Autodesk Inventor part; units mm, degrees
ref_plane "YZ Plane" through (0, 0, 0) normal (1, 0, 0) x (0, 1, 0)
ref_plane "XZ Plane" through (0, 0, 0) normal (0, 1, 0) x (-1, 0, 0)
ref_plane "XY Plane" through (0, 0, 0) normal (0, 0, 1) x (1, 0, 0)
sketch "Sketch1" plane through (0, 0, 0) normal (0, 0, 1) x (1, 0, 0)
  line L0 (21.2725, 0) -> (23.8125, 0)
  line L1 (23.8125, 0) -> (23.8125, 28.3972)
  line L2 (23.8125, 28.3972) -> (6.985, 28.3972)
  line L3 (21.2725, 25.8572) -> (21.2725, 0)
  line L4 (0, -5.6794) -> (0, 34.0766)
  line L5 (6.985, 25.8572) -> (6.985, 28.3972)
  line L6 (6.985, 25.8572) -> (21.2725, 25.8572)
  point P0 (0, 0)
  dimension "d5" = 28.3972
  dimension "d10" = 21.2725
  dimension "d13" = 2.54
  dimension "d22" = 6.985
  dimension "d50" = 2.54
revolve "Revolution1" add sketch "Sketch1" angle 360 about axis through (0, -10, 0) along (0, 1, 0)
sketch "Sketch4" plane through (0, 0, 0) normal (1, 0, 0) x (0, 1, 0)
  circle A0 centre (8.001, 0) radius 1.5875
  point P0 (0, 0)
  dimension "d33" = 3.175
  dimension "d34" = 8.001
extrude "Extrusion2" cut sketch "Sketch4" along normal through all
pattern_circular "Circular Pattern1" count 3 over 360 about axis through (0, 14.1986, 0) along (0, -1, 0) of "Extrusion2"
sketch "Sketch5" plane through (0, 28.3972, 0) normal (0, 1, 0) x (1, 0, 0)
  line L0 (6.985, 7.9248) -> (-6.985, 7.9248)
  line L1 (-6.985, 7.9248) -> (-6.985, -8.5852)
  line L2 (-6.985, -8.5852) -> (6.985, -8.5852)
  line L3 (6.985, -8.5852) -> (6.985, 7.9248)
  line L4 (6.985, 7.9248) -> (-6.985, -8.5852) construction
  line L5 (-6.985, 7.9248) -> (6.985, -8.5852) construction
  circle A0 centre (0, 0) radius 6.985 construction
  point P0 (0, -0.3302)
  dimension "d51" = 13.97
  dimension "d52" = 16.51
  dimension "d56" = 0.3302
extrude "Extrusion3" cut sketch "Sketch5" against normal through all
sketch "Sketch6" plane through (0, 28.3972, 0) normal (0, 1, 0) x (1, 0, 0)
  circle A0 centre (-15.24, -7.62) radius 1.3959
  line L0 (0, 0) -> (-15.24, -7.62) construction
  line L1 (-15.24, -7.62) -> (0, -7.62) construction
  line L2 (0, -7.62) -> (0, 0) construction
  dimension "d59" = 7.62
  dimension "d60" = 15.24
extrude "Extrusion4" cut sketch "Sketch6" against normal through all
properties part number "Gauge Housing"
Verification items for the finished model (mm, model axes). A direction names the side the tool comes from. Give positions to 0.01 mm unless a question says otherwise; leave off trailing zeros. Order: outer loops, then holes, each group sorted by start corner. A loop starts at its lowest first (then second) coordinate and runs counter-clockwise, first axis right, second up. Notation, with made-up numbers: (2.5, -19.5) -> (30.5, -19.5) arc R28 ccw to (30.5, 11.5) -> close; hole circle Ø10 at (16.25, -32.5). An arc over 180 degrees is marked (long way). Answer as CSV lines item,"result".
Q1. Sectioned sample at B-B on z = 0. Record the cut outline in (x, y) (1 decimal).
Solutions:
outline,"(-23.8, 0) -> (-21.3, 0) -> (-21.3, 25.9) -> (-7, 25.9) -> (-7, 28.4) -> (-23.8, 28.4) -> close; (7, 25.9) -> (21.3, 25.9) -> (21.3, 9.6) -> (23.8, 9.6) -> (23.8, 28.4) -> (7, 28.4) -> close; (21.3, 0) -> (23.8, 0) -> (23.8, 6.4) -> (21.3, 6.4) -> close"
Q2. Release check for a two-part mould opening along Z. For faces 5 (the cylindrical face through (-18.897, 14.397, 14.49)), 6 (the flat face through (-9, 0, -20)), 7 (the cylindrical face through (-16.881, 12.748, -12.944)) record: +Z half, -Z half, draft (parallel to the pull), parting line (faces both ways), or undercut.
Solutions:
face 5,"parting line"
face 6,"draft"
face 7,"undercut"
Q3. Sectioned sample at A-A on x = 0. Record the cut outline in (y, z).
Solutions:
outline,"(0, -23.81) -> (28.4, -23.81) -> (28.4, -7.92) -> (25.86, -7.92) -> (25.86, -21.27) -> (0, -21.27) -> close; (0, 21.27) -> (25.86, 21.27) -> (25.86, 8.59) -> (28.4, 8.59) -> (28.4, 23.81) -> (0, 23.81) -> close"
Q4. Sectioned sample at C-C on y = 8.25. Record the cut outline in (x, z) (1 decimal).
Solutions:
outline,"(-13.2, -19.8) -> (-12, -17.6) arc R21.3 cw to (-12, 17.6) -> (-13.2, 19.8) arc R23.8 ccw to start; (-10.5, -21.4) arc R23.8 ccw to (23.8, -1.6) -> (21.2, -1.6) arc R21.3 cw to (-9.2, -19.2) -> close; (-10.5, 21.4) -> (-9.2, 19.2) arc R21.3 cw to (21.2, 1.6) -> (23.8, 1.6) arc R23.8 ccw to start"
Q5. Depth check by flat-ended pin: pin 1 (2 mm diameter, centred on y = 27.5, z = 3.5, fed in from +X); pin 2 (2 mm diameter, centred on y = 27, z = -2, fed in from -X); pin 3 (3.5 mm diameter, centred on x = -15.24, z = 7.62, fed in from -Y). Enter the tip coordinate at first touch or a pass-through.
Solutions:
pin 1,"stops at x = 23.68"
pin 2,"stops at x = -23.79"
pin 3,"stops at y = 25.86"
Q6. Sectioned sample at D-D on z = 5. Record the cut outline in (x, y) (3 decimals), plus the area to 3 significant figures.
Solutions:
outline,"(-23.282, 0) -> (-20.677, 0) -> (-20.677, 25.857) -> (-6.985, 25.857) -> (-6.985, 28.397) -> (-23.282, 28.397) -> close; (6.985, 25.857) -> (20.677, 25.857) -> (20.677, 0) -> (23.282, 0) -> (23.282, 28.397) -> (6.985, 28.397) -> close"
area,"218 mm²"
Q7. Access from +Z, -Z, +X, -X, +Y, -Y to the whole of each face (thin tool, end or side, straight path). Record for faces 1 (the flat face through (-6.985, 27, 0)), 2 (the cylindrical face through (22.495, 6.415, -0.07)), 3 (the flat face through (10, 28.397, 0)), 4 (the flat face through (0, 25.857, 9)).
Solutions:
face 1,"+Y, -Y"
face 2,"+X"
face 3,"+Z, -Z, +X, -X, +Y"
face 4,"-Y"
Q8. Scan lines: probe 1 along Z at (x, y) = (0, 17); probe 2 along Y at (x, z) = (22, 0); probe 3 along X at (y, z) = (26.9, 7.62) (3 decimals). Record each from-to range of solid material in increasing order.
Solutions:
probe 1,"z = -23.81 to -21.27, 21.27 to 23.81"
probe 2,"y = 0 to 6.41, 9.59 to 28.4"
probe 3,"x = -22.56 to -16.636, -13.844 to -6.985, 6.985 to 22.56"
